Part model, mm, in its own coordinate system. A direction names the side the tool comes from. Round coordinates to 2 decimals unless told otherwise and drop trailing zeros. Loops run counter-clockwise (first coordinate to the right, second up) from the corner with the lowest first, then second, coordinate; pieces in that order, holes last. Notation, with made-up numbers: M 20,47.25 L 77,47.25 A37 ccw 77,86.25 Z; hole C 77,82 d4. An arc over 180 degrees is marked long. Put each result on its own line as item: value. Start each with the question number.
1) Probe line 1 along Z through (x, y) = (-33, -29); line 2 along Y through (x, z) = (-17.5, -0.5); line 3 along X through (y, z) = (-1.5, 33.5). List the from-to ranges inside material, lowest first.
2) Slice it at A-A on z = 90. Give the cut face in (x, y), then the cut area to 3 significant figures.
3) Pull direction Z, two halves, no side cores. Call faces 6 (the flat face through (-29, -7, -2)), 7 (the cylindrical face through (2.64, -7.47, 87.07)), 8 (the flat face through (-10, 3.18, 38)): +Z half, -Z half, draft (parallel to the pull), parting line (faces both ways), or undercut.
4) Drop flat-ended pins along their axis: pin 1 Ø1.5 at (x, z) = (-34, -3.5) entering from -Y; pin 2 Ø10 at (y, z) = (-11, 53) entering from +X; pin 3 Ø3 at (y, z) = (-11, 13) entering from -X. Give the stop position or say it passes through.
5) Slice it at C-C on y = -25.5. Give the cut face in (x, z).
6) Which spindle directions (+Z, -Z, +X, -X, +Y, -Y) get a long thin tool onto all of the face, cutting with end or side? Do faces 1 (the flat face through (-32, -8.82, -4)), 2 (the flat face through (-14.57, -3.1, -3.52)), 3 (the flat face through (-16.378, -7, 54)), 4 (the flat face through (3.622, -7, 49)), 5 (the flat face through (-15, -20, 0)). Say none if no direction does.
7) Slice it at D-D on z = 26. Give the cut face in (x, y).
8) Slice it at B-B on z = 38.5. Give the cut face in (x, y), then the cut area to 3 significant figures.
```python
from build123d import *

# Parameters (mm, degrees)
SKETCH_1_W          = 20
SKETCH_1_H          = 20
EXTRUDE_1_DEPTH     = 140
SKETCH_2_R          = 30
SKETCH_2_R_2        = 1.55
EXTRUDE_2_DEPTH     = 5
SKETCH_3_W          = 28.284271248
SKETCH_3_H          = 20
EXTRUDE_3_DEPTH     = 28.28427125
CUT_EXTRUDE_1_DEPTH = 28.28427125
CUT_EXTRUDE_2_DEPTH = 28.28427125
CUT_EXTRUDE_3_DEPTH = 28.28427125
SKETCH_8_R          = 3
CUT_EXTRUDE_4_DEPTH = 2
SKETCH_9_R          = 2
CUT_EXTRUDE_5_DEPTH = 100
CUT_EXTRUDE_6_DEPTH = 3


with BuildPart() as part:
    # 草图1 → 凸台-拉伸1 (new body)
    with BuildSketch(Plane.XY):
        with Locations((-6.377546769, -6.820183169)):
            Rectangle(SKETCH_1_W, SKETCH_1_H)
    extrude(amount=EXTRUDE_1_DEPTH)

    # 草图2 → 凸台-拉伸2 (add)
    with BuildSketch(Plane(origin=(0, 0, 0), x_dir=(-1, 0, 0), z_dir=(0, 0, -1))):
        with Locations((16.377546769, -6.820183169)):
            Circle(SKETCH_2_R)
        with Locations((-6.572126431, 6.429816831)):
            Circle(SKETCH_2_R_2, mode=Mode.SUBTRACT)
        with Locations((16.377546769, 19.679816831)):
            Circle(SKETCH_2_R_2, mode=Mode.SUBTRACT)
        with Locations((39.32721997, 6.429816831)):
            Circle(SKETCH_2_R_2, mode=Mode.SUBTRACT)
        with Locations((39.32721997, -20.070183169)):
            Circle(SKETCH_2_R_2, mode=Mode.SUBTRACT)
        with Locations((16.377546769, -33.320183169)):
            Circle(SKETCH_2_R_2, mode=Mode.SUBTRACT)
        with Locations((-6.572126431, -20.070183169)):
            Circle(SKETCH_2_R_2, mode=Mode.SUBTRACT)
    extrude(amount=EXTRUDE_2_DEPTH)

    # 草图3 → 凸台-拉伸3 (add)
    with BuildSketch(Plane.XY):
        with Locations((-30.519682393, -6.820183169)):
            Rectangle(SKETCH_3_W, SKETCH_3_H)
    extrude(amount=EXTRUDE_3_DEPTH)

    # 草图4 → 切除-拉伸1 (cut)
    with BuildSketch(Plane(origin=(0, 3.179816831, 0), x_dir=(1, 0, 0), z_dir=(0, 1, 0))):
        with BuildLine():
            Line((-44.661818017, -3e-09), (-44.661818017, -28.28427125))
            Line((-44.661818017, -28.28427125), (-16.377546769, -28.28427125))
            ThreePointArc((-16.377546769, -28.28427125), (-24.661818017, -8.28427125), (-44.661818017, -3e-09))
        make_face()
    extrude(amount=-CUT_EXTRUDE_1_DEPTH, mode=Mode.SUBTRACT)

    # 草图6 → 切除-拉伸2 (cut)
    with BuildSketch(Plane(origin=(0, 3.179816831, 0), x_dir=(1, 0, 0), z_dir=(0, 1, 0))):
        Polygon((3.622453231, -140), (3.622453231, -100), (-6.377546769, -100), (-6.377546769, -80), (-16.377546769, -80), (-16.377546769, -100), (-16.377546769, -140), align=None)
    extrude(amount=-CUT_EXTRUDE_2_DEPTH, mode=Mode.SUBTRACT)

    # 草图7 → 切除-拉伸3 (cut)
    with BuildSketch(Plane.ZY.offset(6.377546769)):
        with BuildLine():
            ThreePointArc((91.55, -6.820183169), (90.59315932, -5.388169893), (88.903984489, -5.724167658))
            Line((88.903984489, -5.724167658), (91.096015511, -7.91619868))
            ThreePointArc((91.096015511, -7.91619868), (91.432013275, -7.413342489), (91.55, -6.820183169))
        make_face()
        with BuildLine():
            Line((91.096015511, -7.91619868), (88.903984489, -5.724167658))
            ThreePointArc((88.903984489, -5.724167658), (88.903984489, -7.91619868), (91.096015511, -7.91619868))
        make_face()
    extrude(amount=-CUT_EXTRUDE_3_DEPTH, mode=Mode.SUBTRACT)

    # 草图8 → 切除-拉伸4 (cut)
    with BuildSketch(Plane(origin=(3.622453231, 0, 0), x_dir=(0, 0, -1), z_dir=(1, 0, 0))):
        with Locations(Location((-90, -6.820183169, 0), (0, 0, 90))):
            Circle(SKETCH_8_R)
    extrude(amount=-CUT_EXTRUDE_4_DEPTH, mode=Mode.SUBTRACT)

    # 草图9 → 切除-拉伸5 (cut)
    with BuildSketch(Plane.XY.offset(80)):
        with Locations((-11.377546769, -2.820183169)):
            Circle(SKETCH_9_R)
    extrude(amount=-CUT_EXTRUDE_5_DEPTH, mode=Mode.SUBTRACT)

    # 草图10 → 切除-拉伸6 (cut)
    with BuildSketch(Plane(origin=(0, 0, -5), x_dir=(-1, 0, 0), z_dir=(0, 0, -1))):
        Polygon((16.377546769, -4.820183169), (48.333202205, -4.820183169), (48.333202205, -8.820183169), (16.377546769, -8.820183169), (10.220063838, -4.45167354), (11.377546769, -2.820183169), (12.810373312, -1.424830848), align=None)
    extrude(amount=-CUT_EXTRUDE_6_DEPTH, mode=Mode.SUBTRACT)


solid = part.part
```
Recorded:
1. line 1: z = -5 to 0
1. line 2: y = -36.8 to -34.39, -32.25 to 18.61, 20.75 to 23.16
1. line 3: x = -16.38 to -12.88, -9.88 to 3.62
2. outline: M -6.38,-16.82 L 3.62,-16.82 L 3.62,-9.82 L 1.62,-9.82 L 1.62,-8.37 L -6.38,-8.37 Z; M -6.38,-5.27 L 1.62,-5.27 L 1.62,-3.82 L 3.62,-3.82 L 3.62,3.18 L -6.38,3.18 Z
2. area: 163 mm2
3. face 6: -Z half
3. face 7: undercut
3. face 8: draft
4. pin 1: stops at y = -31.63
4. pin 2: stops at x = 3.62
4. pin 3: stops at x = -21.9
5. outline: M -39.85,-5 L 7.1,-5 L 7.1,0 L -39.85,0 Z
6. face 1: -Z, -X
6. face 2: -Z
6. face 3: +Z, -X, +Y, -Y
6. face 4: +Z, +X, +Y, -Y
6. face 5: +Z, +X
7. outline: M -16.47,-16.82 L 3.62,-16.82 L 3.62,3.18 L -16.47,3.18 Z; hole C -11.38,-2.82 d4
8. outline: M -16.38,-16.82 L 3.62,-16.82 L 3.62,3.18 L -16.38,3.18 Z; hole C -11.38,-2.82 d4
8. area: 387 mm2
